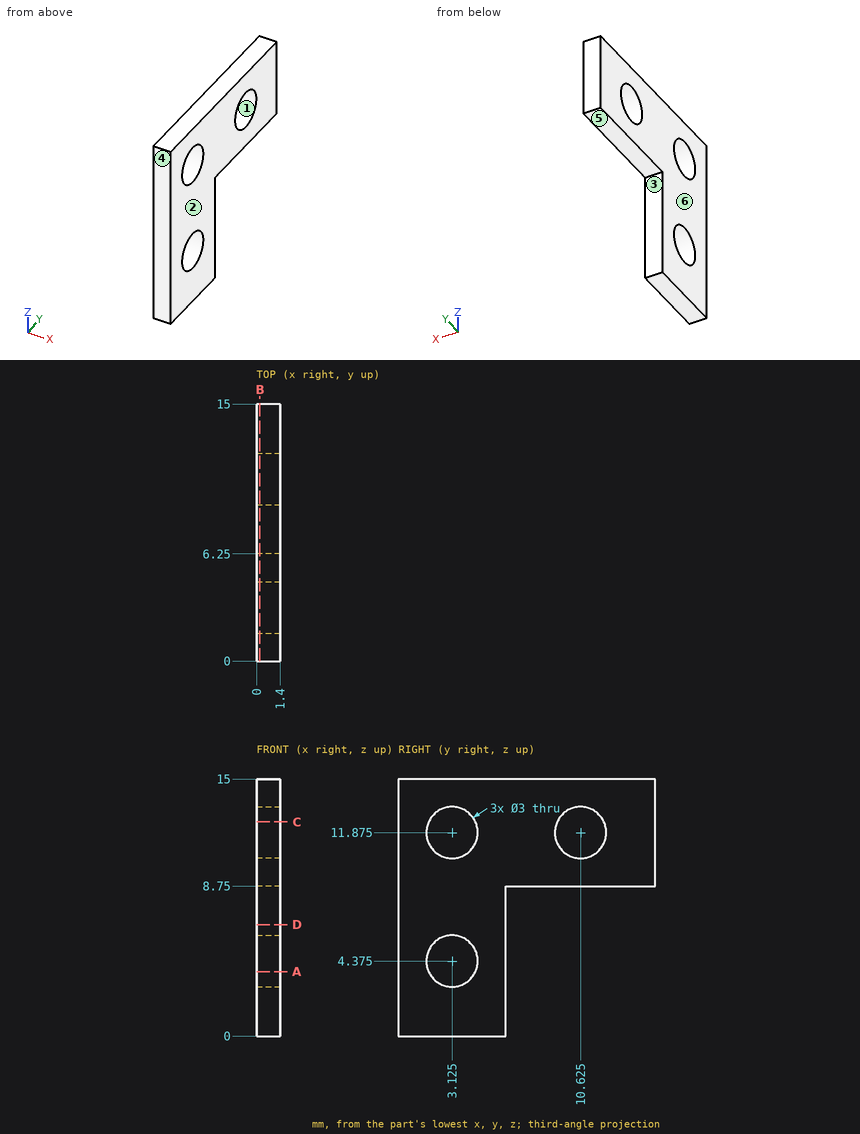
Print and shaded views of the part. All mm, measured from the part's lowest x, y and z. A direction names the side the tool comes from. Give positions to 0.01 mm unless a question says otherwise; leave off trailing zeros. Loops run counter-clockwise (first coordinate to the right, second up) from the corner with the lowest first, then second, coordinate; pieces in that order, holes last. Notation, with made-up numbers: (-22.5, 16) - (-13.5, 16) arc R26 ccw to (-13.5, 43) - close; hole circle Ø9 at (-27.5, 83.5). An arc over 180 degrees is marked (long way). One line per item, written item: value. Start each with the question number.
1. Slice it at D-D (z = 6.5). List the corners of the cut face in (x, y).
2. Slice it at C-C (z = 12.5). List the corners of the cut face in (x, y), plus the area to 3 significant figures.
3. Which spindle directions (+Z, -Z, +X, -X, +Y, -Y) get a long thin tool onto all of the face, cutting with end or side? Do the marked faces 5 and 6. Say none if no direction does.
4. Pull direction Y, two halves, no side cores. Call the marked faces 1, 2, 3 and 4: pulls with the +Y half, pulls with the -Y half, needs draft (parallel to the pull), parting line crosses it, or undercut.
5. Slice it at A-A (z = 3.75). List the corners of the cut face in (x, y), plus the area to 3 significant figures.
6. Slice it at B-B (x = 0.2). List the corners of the cut face in (y, z) (3 decimals).
7. Pin check, flat tip, straight feed: pin 1 (4 mm diameter, centred on y = 10.625, z = 11.875, fed in from -X). Stop position of the tip, or through.
8. Probe L1, parallel to Z at x = 0.65, y = 3; L2, parallel to Z at x = 1.3, y = 2.5; L3, parallel to Y at x = 0.75, z = 7.25. List the from-to ranges inside material, lowest first. Write a range as from..to.
Solution:
1. outline: (0, 0) - (1.4, 0) - (1.4, 6.25) - (0, 6.25) - close
2. outline: (0, 0) - (1.4, 0) - (1.4, 1.76) - (0, 1.76) - close; (0, 4.49) - (1.4, 4.49) - (1.4, 9.26) - (0, 9.26) - close; (0, 11.99) - (1.4, 11.99) - (1.4, 15) - (0, 15) - close
2. area: 13.4 mm^2
3. face 5: -Z, +X, -X, +Y
3. face 6: +Z, -Z, -X, +Y, -Y
4. face 1: undercut
4. face 2: needs draft
4. face 3: pulls with the +Y half
4. face 4: pulls with the -Y half
5. outline: (0, 0) - (1.4, 0) - (1.4, 1.76) - (0, 1.76) - close; (0, 4.49) - (1.4, 4.49) - (1.4, 6.25) - (0, 6.25) - close
5. area: 4.93 mm^2
6. outline: (0, 0) - (6.25, 0) - (6.25, 8.75) - (15, 8.75) - (15, 15) - (0, 15) - close; hole circle Ø3 at (3.125, 4.375); hole circle Ø3 at (3.125, 11.875); hole circle Ø3 at (10.625, 11.875)
7. pin 1: stops at x = 0
8. L1: z = 0..2.88, 5.87..10.38, 13.37..15
8. L2: z = 0..3.01, 5.74..10.51, 13.24..15
8. L3: y = 0..6.25
